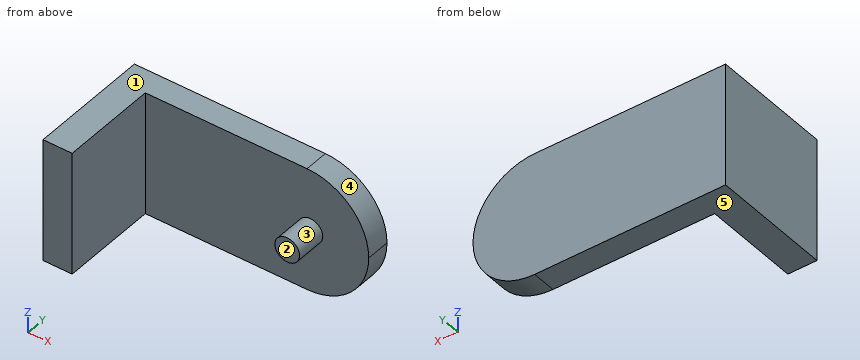
from build123d import *

# Parameters (mm, degrees)
F1_DEPTH = 12.7
F2_R     = 1.27
F3_DEPTH = 3.175
F4_R     = 6.34999


# Not quite as in the source:
# - a fillet or chamfer is up to 0.001 mm smaller than in the source, because OpenCascade refuses the exact size


with BuildPart() as f1:
    # F0 (on Top) → F1 (new body)
    with BuildSketch(Plane.XY):
        Polygon((0, -12.5), (3, -12.5), (3, -2.5), (26, -2.5), (26, 0), (0, 0), align=None)
    extrude(amount=F1_DEPTH)

    # F2 (on face) → F3 (join)
    with BuildSketch(Plane.XZ.offset(2.5)):
        with Locations((20, 6.35)):
            Circle(F2_R)
    extrude(amount=F3_DEPTH)

    # F4 (radius 6.35 in the source; OpenCascade refuses exactly that, so slightly less here)
    f4_edges = [f1.edges().sort_by_distance(p)[0] for p in [
        (26, -1.25, 12.7),
        (26, -1.25, 0),
    ]]
    fillet(f4_edges, radius=F4_R)


solid = f1.part
Geometry: final body of the model. Coordinates: model frame, mm. Face numbers are marked on the shaded views. A direction names the side the tool comes from. Give positions to 0.01 mm unless a question says otherwise; leave off trailing zeros. Order: outer loops, then holes, each group sorted by start corner. A loop starts at its lowest first (then second) coordinate and runs counter-clockwise, first axis right, second up. Notation, with made-up numbers: (-7.5, 81) -> (24.5, 81) arc R22 ccw to (24.5, 98) -> close; hole circle Ø8 at (47, -6). An arc over 180 degrees is marked (long way). Answer as a JSON object with one key per item and string values.
Q1. Draft query along X for the marked faces 3, 4 and 5. Return one class per face: released by +X, released by -X, zero draft, split by the parting line, or undercut.
Entries:
{"face 3": "undercut", "face 4": "released by +X", "face 5": "zero draft"}
Q2. Section C-C (y = -7.75). Output: boundary loops of the cut face in (x, z).
Entries:
{"outline": "(0, 0) -> (3, 0) -> (3, 12.7) -> (0, 12.7) -> close"}
Q3. Section B-B (z = 7.25). Output: boundary loops of the cut face in (x, y) (3 decimals), plus the area to 3 significant figures.
Entries:
{"outline": "(0, -12.5) -> (3, -12.5) -> (3, -2.5) -> (19.104, -2.5) -> (19.104, -5.675) -> (20.896, -5.675) -> (20.896, -2.5) -> (25.936, -2.5) -> (25.936, 0) -> (0, 0) -> close", "area": "101 mm^2"}
Q4. Access query for the marked faces 1 and 2. Directions: +Z, -Z, +X, -X, +Y, -Y. A direction counts if a zero-diameter tool reaches every point of the face in a straight line with its end or side. Return the directions, or none.
Entries:
{"face 1": "+Z, +X, -X, +Y, -Y", "face 2": "+Z, -Z, +X, -Y"}
Q5. Section D-D (x = 20). Output: boundary loops of the cut face in (y, z) (3 decimals).
Entries:
{"outline": "(-5.675, 5.08) -> (-2.5, 5.08) -> (-2.5, 0.01) -> (0, 0.01) -> (0, 12.69) -> (-2.5, 12.69) -> (-2.5, 7.62) -> (-5.675, 7.62) -> close"}
Q6. Material intervals for probe 1 along X at (y, z) = (-3.5, 9.5); probe 2 along Y at (x, z) = (4, 12); probe 3 along Y at (x, z) = (19.5, 6) (3 decimals), sorted ascending.
Entries:
{"probe 1": "x = 0 to 3", "probe 2": "y = -2.5 to 0", "probe 3": "y = -5.675 to 0"}
Q7. First-contact query: pin 1 (2 mm diameter, centred on x = 20, z = 7, fed in from -Y) (3 decimals); pin 2 (1.5 mm diameter, centred on y = -3, z = 8, fed in from +X). Flat tips, straight axial feed; report the tip coordinate or a pass-through.
Entries:
{"pin 1": "stops at y = -5.675", "pin 2": "stops at x = 25.91"}
Q8. Section A-A (y = -3.75). Output: boundary loops of the cut face in (x, z), plus the area to 3 significant figures.
Entries:
{"outline": "(0, 0) -> (3, 0) -> (3, 12.7) -> (0, 12.7) -> close; circle Ø2.54 at (20, 6.35)", "area": "43.2 mm^2"}
